Verification items for the finished model (mm, model axes). Face numbers are marked on the shaded views. A direction names the side the tool comes from. Give positions to 0.01 mm unless a question says otherwise; leave off trailing zeros. Order: outer loops, then holes, each group sorted by start corner. A loop starts at its lowest first (then second) coordinate and runs counter-clockwise, first axis right, second up.
(1) Mould release check, pull along Y, two halves, no side actions. Record for the marked faces 3, 4 and 5: pulls with the +Y half, pulls with the -Y half, needs draft (parallel to the pull), parting line crosses it, or undercut.
(2) Scan lines: L1, parallel to X at y = -21.5, z = 2.7; L2, parallel to X at y = -21, z = 2.2; L3, parallel to X at y = -7, z = 2.65. Record each from-to range of solid material in increasing order.
(3) Sectioned sample at B-B on y = -22. Record the cut outline in (x, z) (3 decimals).
(4) Sectioned sample at C-C on z = 1.15. Count the separate pieces of the cut face and the enclosed holes in it, plus the area to 3 significant figures.
(5) Sectioned sample at D-D on y = 6.5. Record the cut outline in (x, z) (3 decimals).
(6) Sectioned sample at A-A on x = 0. Record the cut outline in (y, z) (3 decimals), plus the area to 3 significant figures.
(7) Gauge pin test, flat end, axial feed: pin 1 (2.5 mm diameter, centred on x = -6.5, y = 0, fed in from -Z). Record the tip position at first contact, or that the pin passes through.
(8) Access from +Z, -Z, +X, -X, +Y, -Y to the whole of each face (thin tool, end or side, straight path). Record for the marked faces 1 and 2.
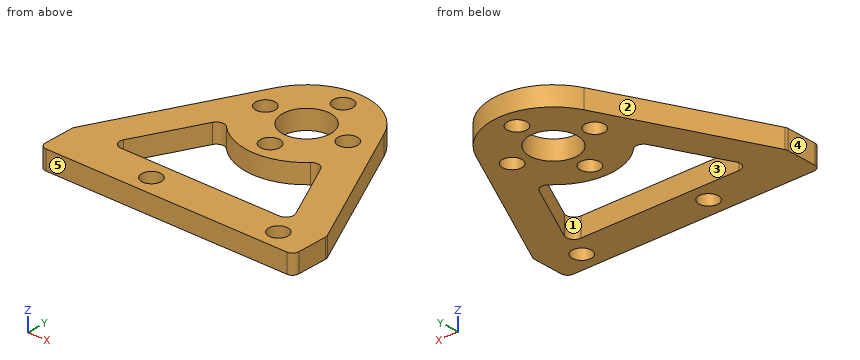
```python
from build123d import *

# Parameters (mm, degrees)
SKETCH_1_R          = 1.525
SKETCH_1_R_2        = 3.75
EXTRUDE_1_DEPTH     = 3
FILLET_1_R          = 1
SKETCH_2_R          = 1.515
CUT_EXTRUDE_1_DEPTH = 10
CUT_EXTRUDE_2_DEPTH = 10
FILLET_2_R          = 1.2


with BuildPart() as part:
    # 草图1 → 凸台-拉伸1 (new body)
    with BuildSketch(Plane.XY):
        with BuildLine():
            Line((-20, -25), (20, -25))
            Line((20, -25), (20, -19))
            Line((20, -19), (8.514771251, 4.212917106))
            ThreePointArc((8.514771251, 4.212917106), (0, 9.5), (-8.514771251, 4.212917106))
            Line((-8.514771251, 4.212917106), (-20, -19))
            Line((-20, -19), (-20, -25))
        make_face()
        with Locations((0, 6.5)):
            Circle(SKETCH_1_R, mode=Mode.SUBTRACT)
        with Locations((6.5, 0)):
            Circle(SKETCH_1_R, mode=Mode.SUBTRACT)
        with Locations((0, -6.5)):
            Circle(SKETCH_1_R, mode=Mode.SUBTRACT)
        with Locations((-6.5, 0)):
            Circle(SKETCH_1_R, mode=Mode.SUBTRACT)
        Circle(SKETCH_1_R_2, mode=Mode.SUBTRACT)
    extrude(amount=EXTRUDE_1_DEPTH)

    # 圆角1
    fillet_1_edges = [part.edges().sort_by_distance(p)[0] for p in [
        (20, -25, 1.5),
        (-20, -25, 1.5),
        (-20, -19, 1.5),
        (20, -19, 1.5),
    ]]
    fillet(fillet_1_edges, radius=FILLET_1_R)

    # 草图2 → 切除-拉伸1 (cut)
    with BuildSketch(Plane(origin=(0, 0, 0), x_dir=(-1, 0, 0), z_dir=(0, 0, -1))):
        with Locations((-15, -22)):
            Circle(SKETCH_2_R)
        with Locations((5, -22)):
            Circle(SKETCH_2_R)
    extrude(amount=-CUT_EXTRUDE_1_DEPTH, mode=Mode.SUBTRACT)

    # 草图3 → 切除-拉伸2 (cut)
    with BuildSketch(Plane(origin=(0, 0, 0), x_dir=(-1, 0, 0), z_dir=(0, 0, -1))):
        with BuildLine():
            Line((-7.743606738, -5.50332215), (-14.421459062, -19))
            Line((-14.421459062, -19), (14.421459062, -19))
            Line((14.421459062, -19), (7.743606738, -5.50332215))
            ThreePointArc((7.743606738, -5.50332215), (0, -9.5), (-7.743606738, -5.50332215))
        make_face()
    extrude(amount=-CUT_EXTRUDE_2_DEPTH, mode=Mode.SUBTRACT)

    # 圆角2
    fillet_2_edges = [part.edges().sort_by_distance(p)[0] for p in [
        (7.743606738, -5.50332215, 1.5),
        (-7.743606738, -5.50332215, 1.5),
        (-14.421459062, -19, 1.5),
        (14.421459062, -19, 1.5),
    ]]
    fillet(fillet_2_edges, radius=FILLET_2_R)


solid = part.part
```
Ans:
1. face 3: undercut
1. face 4: needs draft
1. face 5: pulls with the -Y half
2. L1: x = -20 to -6.43, -3.57 to 13.57, 16.43 to 20
2. L2: x = -20 to -6.14, -3.86 to 13.86, 16.14 to 20
2. L3: x = -14.06 to -8.47, -6.42 to -1.44, 1.44 to 6.42, 8.47 to 14.06
3. outline: (-20, 0) - (-6.515, 0) - (-6.515, 3) - (-20, 3) - close; (-3.485, 0) - (13.485, 0) - (13.485, 3) - (-3.485, 3) - close; (16.515, 0) - (20, 0) - (20, 3) - (16.515, 3) - close
4. separate pieces: 1
4. enclosed holes: 8
4. area: 625 mm2
5. outline: (-6.928, 0) - (-1.525, 0) - (-1.525, 3) - (-6.928, 3) - close; (1.525, 0) - (6.928, 0) - (6.928, 3) - (1.525, 3) - close
6. outline: (-25, 0) - (-19, 0) - (-19, 3) - (-25, 3) - close; (-9.5, 0) - (-8.025, 0) - (-8.025, 3) - (-9.5, 3) - close; (-4.975, 0) - (-3.75, 0) - (-3.75, 3) - (-4.975, 3) - close; (3.75, 0) - (4.975, 0) - (4.975, 3) - (3.75, 3) - close; (8.025, 0) - (9.5, 0) - (9.5, 3) - (8.025, 3) - close
6. area: 34.2 mm2
7. pin 1: passes through
8. face 1: +Z, -Z
8. face 2: +Z, -Z, -X, +Y
